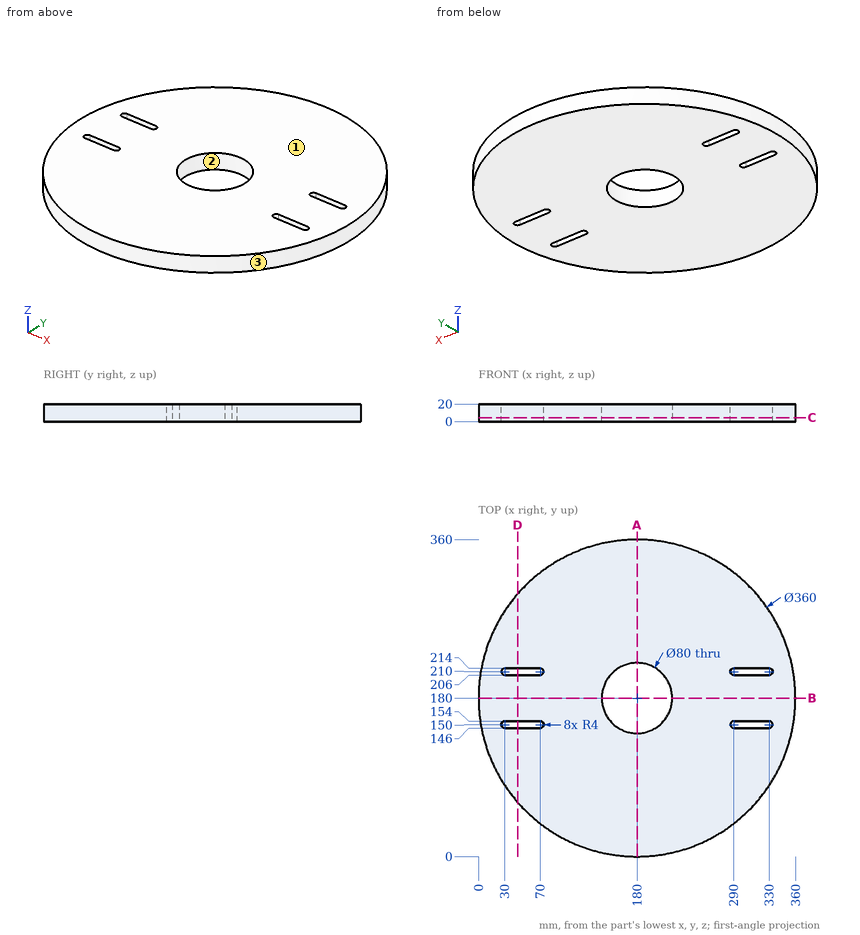
For this review, use the dimensioned drawing (mm, ordinates from the lowest corner) and the shaded views. Coordinates: 2 decimals unless noted, no trailing zeros. Write each loop counter-clockwise with the first axis right and the second up, starting at its lowest first coordinate (ties: lowest second). Pieces come first, ordered by that corner, then holes. Notation, with made-up numbers: (63.25, 69) -> (105.25, 69) arc R19 cw to (105.25, 104) -> close; hole circle Ø2 at (65, 82.25). An arc over 180 degrees is marked (long way). Write each question's results on one line, items separated by ' | '. Start each with the question number.
(1) Take a section at A-A on x = 180. Write out the cut boundary in (y, z), and give its area (3 significant figures).
(2) For line 1 along Y through (x, z) = (180, 13.25); line 2 along Y through (x, z) = (72, 16.25); line 3 along Y through (x, z) = (44.5, 16), list the stretches that pass through material, from the lowest coordinate up. Write a range as from..to.
(3) Clearance check with flat-ended pins moving along their axes: P1, Ø6, axis at x = 44, z = 9, coming from the -Y side; P2, Ø6, axis at y = 291.5, z = 11.5, coming from the -X side; P3, Ø10, axis at x = 307.5, z = 13.5, coming from the +Y side; P4, Ø5, axis at x = 38.5, y = 247, coming from the -Z side. State where each tip first meets the part, or that it passes through.
(4) The part is to be moulded in two halves that separate along X. For the marked faces 1, 2 and 3, say which applies: pulls with the +X half, pulls with the -X half, needs draft (parallel to the pull), parting line crosses it, or undercut.
(5) Take a section at C-C on z = 4.5. Write out the cut boundary in (x, y), and give its area (3 significant figures).
(6) Take a section at D-D on x = 44.5. Write out the cut boundary in (y, z).
Results found:
1) outline: (0, 0) -> (140, 0) -> (140, 20) -> (0, 20) -> close; (220, 0) -> (360, 0) -> (360, 20) -> (220, 20) -> close | area: 5,600 mm2
2) line 1: y = 0..140, 220..360 | line 2: y = 36..146.54, 153.46..206.54, 213.46..324 | line 3: y = 61.51..146, 154..206, 214..298.49
3) P1: stops at y = 58.71 | P2: stops at x = 36.38 | P3: stops at y = 311.89 | P4: stops at z = 0
4) face 1: needs draft | face 2: undercut | face 3: parting line crosses it
5) outline: circle Ø360 at (180, 180); hole (30, 146) -> (70, 146) arc R4 ccw to (70, 154) -> (30, 154) arc R4 ccw to start; hole (30, 206) -> (70, 206) arc R4 ccw to (70, 214) -> (30, 214) arc R4 ccw to start; hole circle Ø80 at (180, 180); hole (290, 146) -> (330, 146) arc R4 ccw to (330, 154) -> (290, 154) arc R4 ccw to start; hole (290, 206) -> (330, 206) arc R4 ccw to (330, 214) -> (290, 214) arc R4 ccw to start | area: 95,300 mm2
6) outline: (61.51, 0) -> (146, 0) -> (146, 20) -> (61.51, 20) -> close; (154, 0) -> (206, 0) -> (206, 20) -> (154, 20) -> close; (214, 0) -> (298.49, 0) -> (298.49, 20) -> (214, 20) -> close
